Source: CAD feature listing. Evaluate the final solid. Frame: model axes, mm. A direction names the side the tool comes from. Round coordinates to 2 decimals unless told otherwise and drop trailing zeros. Loops run counter-clockwise (first coordinate to the right, second up) from the corner with the lowest first, then second, coordinate; pieces in that order, holes last.
(1) Section C-C, the plane z = 23. Return the cut outline in (x, y), plus the area to 3 significant figures.
(2) Section D-D, the plane x = 63. Return the cut outline in (y, z), plus the area to 3 significant figures.
(3) First-contact query: pin 1 Ø4 at (y, z) = (3, 20.5) entering from -X; pin 2 Ø5 at (x, z) = (63, 33) entering from +Y; pin 3 Ø2 at (x, y) = (51, 7) entering from +Z. Flat tips, straight axial feed; report the tip coordinate or a pass-through.
(4) Section B-B, the plane y = 36.5. Return the cut outline in (x, z), plus the area to 3 significant figures.
(5) Section A-A, the plane x = 37.5. Return the cut outline in (y, z).
(6) Material intervals for probe 1 along Z at (x, y) = (63, 2); probe 2 along X at (y, z) = (37, 9.5); probe 3 along Y at (x, z) = (77.6, 20), sorted ascending.
(7) Set-up query: faces 4 (the flat face through (40, 5, 29)), 5 (the flat face through (43, 4, 0)), 6 (the flat face through (26, 3, 20)). Return all of +Z, -Z, +X, -X, +Y, -Y with unobstructed straight access to the full face (end or side cutting, diameter ignored); none if empty.
(8) Mould query, pull axis Z, two halves, no side actions, for faces 1 (the flat face through (77, 45, 20)), 2 (the flat face through (43, 4, 40)), 3 (the flat face through (40, 3, 12.5)). Classes: pulls with the +Z half, pulls with the -Z half, needs draft (parallel to the pull), parting line crosses it, or undercut.
Autodesk Inventor part; units mm, degrees
ref_plane "YZ Plane" through (0, 0, 0) normal (1, 0, 0) x (0, 1, 0)
ref_plane "XZ Plane" through (0, 0, 0) normal (0, 1, 0) x (-1, 0, 0)
ref_plane "XY Plane" through (0, 0, 0) normal (0, 0, 1) x (1, 0, 0)
sketch "Sketch1" plane through (0, 0, 0) normal (0, 0, 1) x (1, 0, 0)
  line L0 (0, 0) -> (0, 45)
  line L1 (0, 45) -> (5, 45)
  line L2 (5, 45) -> (5, 5)
  line L3 (5, 5) -> (75, 5)
  line L4 (75, 5) -> (75, 45)
  line L5 (75, 45) -> (80, 45)
  line L6 (80, 45) -> (80, 0)
  line L7 (80, 0) -> (0, 0)
  dimension "d0" = 45
  dimension "d1" = 5
  dimension "d2" = 40
  dimension "d3" = 70
  dimension "d4" = 40
  dimension "d5" = 5
  dimension "d6" = 45
extrude "Extrusion1" add sketch "Sketch1" along normal blind 40
sketch "Sketch2" plane through (80, 0, 0) normal (1, 0, 0) x (0, 0, -1)
  circle A0 centre (-20, 30) radius 5
  line L0 (0, 45) -> (-40, 45)
  line L1 (0, 0) -> (0, 45)
  dimension "d9" = 10
  dimension "d10" = 15
  dimension "d11" = 20
extrude "Extrusion2" cut sketch "Sketch2" against normal through all
sketch "Sketch3" plane through (5, 5, 0) normal (0, 1, 0) x (1, 0, 0)
  line L0 (21, -12.5) -> (49, -12.5)
  line L1 (49, -12.5) -> (49, -27.5)
  line L2 (49, -27.5) -> (21, -27.5)
  line L3 (21, -27.5) -> (21, -12.5)
  line L4 (21, -12.5) -> (49, -27.5) construction
  line L5 (49, -12.5) -> (21, -27.5) construction
  line L6 (70, 0) -> (0, 0)
  line L7 (0, 0) -> (0, -40)
  point P0 (-5, 0)
  point P1 (35, -20)
  dimension "d14" = 28
  dimension "d15" = 15
  dimension "d16" = 20
  dimension "d17" = 35
extrude "Extrusion3" cut sketch "Sketch3" against normal blind 10
sketch "Sketch4" plane through (5, 5, 0) normal (0, 1, 0) x (1, 0, 0)
  circle A0 centre (12, -18.4275) radius 3.625
  circle A1 centre (58, -18.4275) radius 3.625
  line L0 (21, -27.5) -> (21, -12.5)
  line L1 (49, -12.5) -> (49, -27.5)
  point P0 (-5, 0)
  dimension "d20" = 7.25
  dimension "d21" = 7.25
  dimension "d22" = 9
  dimension "d23" = 9
extrude "Extrusion4" cut sketch "Sketch4" against normal blind 2.1735 draft -45
sketch "Sketch5" plane through (17, 2.8265, 18.4275) normal (0, 1, 0) x (1, 0, 0)
  circle A0 centre (0, 0) radius 1.4515
  circle A1 centre (46, 0) radius 1.4515
  line L0 (37, 5.9275) -> (37, -9.0725)
  point P0 (-17, 18.4275)
  dimension "d26" = 2.903
  dimension "d27" = 9
extrude "Extrusion5" cut sketch "Sketch5" against normal through all
properties part number "base and 1st arm link"
Output values:
1. outline: (0, 0) - (26, 0) - (26, 5) - (5, 5) - (5, 26) - (0, 26) - close; (0, 34) - (5, 34) - (5, 45) - (0, 45) - close; (54, 0) - (80, 0) - (80, 26) - (75, 26) - (75, 5) - (54, 5) - close; (75, 34) - (80, 34) - (80, 45) - (75, 45) - close
1. area: 580 mm2
2. outline: (0, 0) - (5, 0) - (5, 14.8) - (2.83, 16.98) - (0, 16.98) - close; (0, 19.88) - (2.83, 19.88) - (5, 22.05) - (5, 40) - (0, 40) - close
2. area: 181 mm2
3. pin 1: stops at x = 0
3. pin 2: stops at y = 5
3. pin 3: passes through
4. outline: (0, 0) - (5, 0) - (5, 40) - (0, 40) - close; (75, 0) - (80, 0) - (80, 40) - (75, 40) - close
4. area: 400 mm2
5. outline: (0, 0) - (5, 0) - (5, 12.5) - (0, 12.5) - close; (0, 27.5) - (5, 27.5) - (5, 40) - (0, 40) - close
6. probe 1: z = 0 to 16.98, 19.88 to 40
6. probe 2: x = 0 to 5, 75 to 80
6. probe 3: y = 0 to 25, 35 to 45
7. face 4: +Z, -Z, +Y
7. face 5: -Z, +X, -X, +Y, -Y
7. face 6: +Y, -Y
8. face 1: needs draft
8. face 2: pulls with the +Z half
8. face 3: undercut
